The listing builds one solid part. Answer for the finished solid, in the listing's coordinates (mm). Face numbers are marked on the shaded views. A direction names the side the tool comes from. Coordinates: 2 decimals unless noted, no trailing zeros. Write each loop counter-clockwise with the first axis right and the second up, starting at its lowest first coordinate (ties: lowest second). Pieces come first, ordered by that corner, then holes.
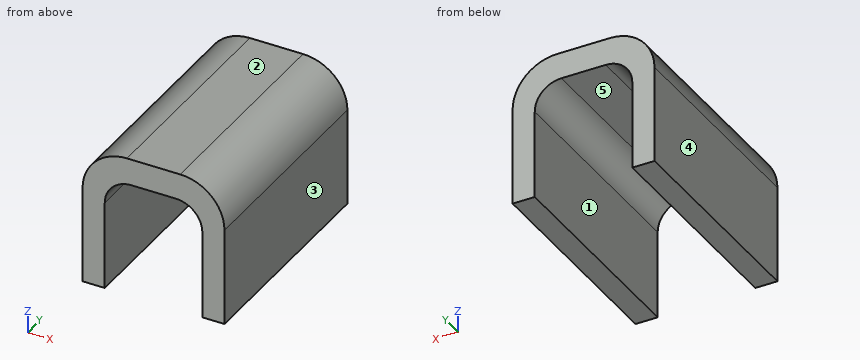
from build123d import *

# Parameters (mm, degrees)
SKETCH_1_W      = 2.5
SKETCH_1_H      = 13
SKETCH_1_W_2    = 16
SKETCH_1_H_2    = 3
EXTRUDE_1_DEPTH = 25
FILLET_1_R      = 3
FILLET_2_R      = 5


with BuildPart() as part:
    # 草图1 → 凸台-拉伸1 (new body)
    with BuildSketch(Plane(origin=(0, 0, 0), x_dir=(1, 0, 0), z_dir=(0, 1, 0))):
        with Locations((6.75, 8)):
            Rectangle(SKETCH_1_W, SKETCH_1_H)
        Rectangle(SKETCH_1_W_2, SKETCH_1_H_2)
        with Locations((-6.75, 8)):
            Rectangle(SKETCH_1_W, SKETCH_1_H)
    extrude(amount=EXTRUDE_1_DEPTH)

    # 圆角1
    fillet_1_edges = [part.edges().sort_by_distance(p)[0] for p in [
        (-5.5, 12.5, -1.5),
        (5.5, 12.5, -1.5),
    ]]
    fillet(fillet_1_edges, radius=FILLET_1_R)

    # 圆角2
    fillet_2_edges = [part.edges().sort_by_distance(p)[0] for p in [
        (8, 12.5, 1.5),
        (-8, 12.5, 1.5),
    ]]
    fillet(fillet_2_edges, radius=FILLET_2_R)


solid = part.part
Q1. Which of the six approach directions +Z, -Z, +X, -X, +Y, -Y give full straight-line access (tool end or side, diameter ignored) to the marked faces 1 and 2?
Answers below:
face 1: -Z, +Y, -Y
face 2: +Z, +X, -X, +Y, -Y
Q2. The part is cut by section B-B, the plane y = 9. Write down the section's boundary in (x, z), then the cut area to 3 significant figures.
Answers below:
outline: (-8, -14.5) - (-5.5, -14.5) - (-5.5, -4.5) arc R3 cw to (-2.5, -1.5) - (2.5, -1.5) arc R3 cw to (5.5, -4.5) - (5.5, -14.5) - (8, -14.5) - (8, -3.5) arc R5 ccw to (3, 1.5) - (-3, 1.5) arc R5 ccw to (-8, -3.5) - close
area: 106 mm2
Q3. Determine the mould class of the marked faces 3, 4 and 5 for opening direction X: released by +X, released by -X, zero draft, split by the parting line, or undercut.
Answers below:
face 3: released by +X
face 4: released by -X
face 5: undercut
Q4. Find the intervals of material crossed by probe 1 along X at (y, z) = (11, -12); probe 2 along Z at (x, y) = (0.5, 6); probe 3 along Z at (x, y) = (-7, 12.5), in increasing order.
Answers below:
probe 1: x = -8 to -5.5, 5.5 to 8
probe 2: z = -1.5 to 1.5
probe 3: z = -14.5 to -0.5
Q5. Given pin 1 (4 mm diameter, centred on x = -5, z = -12, fed in from -Y); pin 2 (5.5 mm diameter, centred on x = -1, y = 16.5, fed in from -Z), each flat-ended and moving along its own axis, determine where each tip first touches the part or whether it passes through.
Answers below:
pin 1: stops at y = 0
pin 2: stops at z = -1.77
Q6. The part is cut by section D-D, the plane z = -2.5. Write down the section's boundary in (x, y), then the cut area to 3 significant figures.
Answers below:
outline: (-7.9, 0) - (-4.74, 0) - (-4.74, 25) - (-7.9, 25) - close; (4.74, 0) - (7.9, 0) - (7.9, 25) - (4.74, 25) - close
area: 158 mm2
Q7. The part is cut by section C-C, the plane x = -2. Write down the section's boundary in (y, z), then the cut area to 3 significant figures.
Answers below:
outline: (0, -1.5) - (25, -1.5) - (25, 1.5) - (0, 1.5) - close
area: 75.0 mm2
Q8. The part is cut by section A-A, the plane z = -10.5. Write down the section's boundary in (x, y), then the cut area to 3 significant figures.
Answers below:
outline: (-8, 0) - (-5.5, 0) - (-5.5, 25) - (-8, 25) - close; (5.5, 0) - (8, 0) - (8, 25) - (5.5, 25) - close
area: 125 mm2
